Design review of the part built by this model. Coordinates are the model's own, in mm. Face numbers are marked on the shaded views. A direction names the side the tool comes from. Round coordinates to 2 decimals unless told otherwise and drop trailing zeros. Write each loop counter-clockwise with the first axis right and the second up, starting at its lowest first coordinate (ties: lowest second). Pieces come first, ordered by that corner, then holes. Notation, with made-up numbers: M 61,8.5 L 71,8.5 A23 cw 71,32.5 Z; hole C 83,-37 d3. An arc over 180 degrees is marked long. Use CSV: the item, a comma, the result in double quotes.
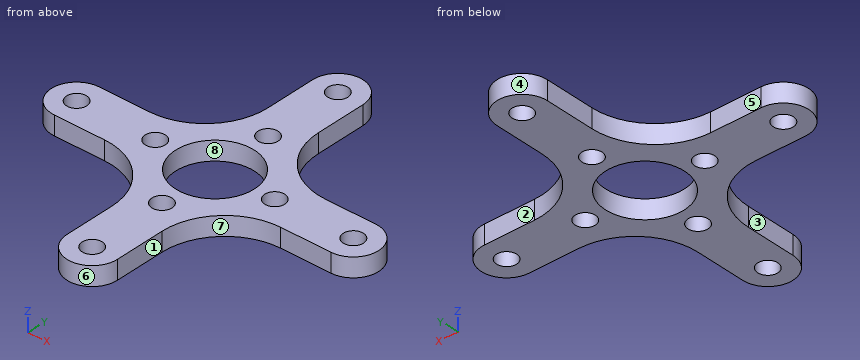
from build123d import *

# Parameters (mm, degrees)
SKETCH_1_R      = 6.25
SKETCH_1_R_2    = 1.6
EXTRUDE_1_DEPTH = 1.5


with BuildPart() as part:
    # Эскиз1 → Бобышка-Вытянуть1 (new body, symmetric)
    with BuildSketch(Plane.XY):
        with BuildLine():
            Line((-22, 4), (-14, 4))
            ThreePointArc((-14, 4), (-6.928932188, 6.928932188), (-4, 14))
            Line((-4, 14), (-4, 22))
            ThreePointArc((-4, 22), (0, 26), (4, 22))
            Line((4, 22), (4, 14))
            ThreePointArc((4, 14), (6.928932188, 6.928932188), (14, 4))
            Line((14, 4), (22, 4))
            ThreePointArc((22, 4), (26, 0), (22, -4))
            Line((22, -4), (14, -4))
            ThreePointArc((14, -4), (6.928932188, -6.928932188), (4, -14))
            Line((4, -14), (4, -22))
            ThreePointArc((4, -22), (0, -26), (-4, -22))
            Line((-4, -22), (-4, -14))
            ThreePointArc((-4, -14), (-6.928932188, -6.928932188), (-14, -4))
            Line((-14, -4), (-22, -4))
            ThreePointArc((-22, -4), (-26, 0), (-22, 4))
        make_face()
        Circle(SKETCH_1_R, mode=Mode.SUBTRACT)
        with Locations((-9.5, 0)):
            Circle(SKETCH_1_R_2, mode=Mode.SUBTRACT)
        with Locations((-22, 0)):
            Circle(SKETCH_1_R_2, mode=Mode.SUBTRACT)
        with Locations((0, 9.5)):
            Circle(SKETCH_1_R_2, mode=Mode.SUBTRACT)
        with Locations((0, 22)):
            Circle(SKETCH_1_R_2, mode=Mode.SUBTRACT)
        with Locations((9.5, 0)):
            Circle(SKETCH_1_R_2, mode=Mode.SUBTRACT)
        with Locations((22, 0)):
            Circle(SKETCH_1_R_2, mode=Mode.SUBTRACT)
        with Locations((0, -22)):
            Circle(SKETCH_1_R_2, mode=Mode.SUBTRACT)
        with Locations((0, -9.5)):
            Circle(SKETCH_1_R_2, mode=Mode.SUBTRACT)
    extrude(amount=EXTRUDE_1_DEPTH, both=True)


solid = part.part
1) Add section C-C on y = 9.5. Write out the cut boundary in (x, z), then the cut area to 3 significant figures.
Answers:
outline,"M -5.07,-1.5 L -1.6,-1.5 L -1.6,1.5 L -5.07,1.5 Z; M 1.6,-1.5 L 5.07,-1.5 L 5.07,1.5 L 1.6,1.5 Z"
area,"20.8 mm²"
2) Wall thickness on line 1 along Y through (x, z) = (0, -0.6); line 2 along Y through (x, z) = (-22, 1.4); line 3 along X through (y, z) = (-1, -0.8): over which ranges is each line inside the solid? List them lowest first. Write a range as [from, to].
Answers:
line 1,"[-26, -23.6], [-20.4, -11.1], [-7.9, -6.25], [6.25, 7.9], [11.1, 20.4], [23.6, 26]"
line 2,"[-4, -1.6], [1.6, 4]"
line 3,"[-25.87, -23.25], [-20.75, -10.75], [-8.25, -6.17], [6.17, 8.25], [10.75, 20.75], [23.25, 25.87]"
3) Add section D-D on x = -9. Write out the cut boundary in (y, z), then the cut area to 3 significant figures.
Answers:
outline,"M -5.34,-1.5 L -1.52,-1.5 L -1.52,1.5 L -5.34,1.5 Z; M 1.52,-1.5 L 5.34,-1.5 L 5.34,1.5 L 1.52,1.5 Z"
area,"22.9 mm²"
4) Machinability: for the marked faces 1, 2, 3, 4 and 5, which of the approach directions +Z, -Z, +X, -X, +Y, -Y give a long, thin tool a straight path to every point of the face, cutting with its end or side? Answer none if there is none.
Answers:
face 1,"+Z, -Z, +X, -Y"
face 2,"+Z, -Z, +X, +Y"
face 3,"+Z, -Z, -X, -Y"
face 4,"+Z, -Z, +Y"
face 5,"+Z, -Z, -X, +Y"
5) Add section B-B on z = -0.7. Give the number of separate pieces and of enclosed holes in the cut face, then the cut area to 3 significant figures.
Answers:
separate pieces,"1"
enclosed holes,"9"
area,"639 mm²"
6) For pin 1 Ø1.5 at (y, z) = (-17, 0) entering from +X; pin 2 Ø0.9 at (y, z) = (16, 0) entering from -X; pin 3 Ø1.5 at (x, z) = (16.5, 0) entering from +Y; pin 4 Ø3 at (x, y) = (9.5, 0) entering from +Z (3 decimals), all flat-tipped, find the tip position at first contact; note any pin that passes through.
Answers:
pin 1,"x = 4"
pin 2,"x = -4"
pin 3,"y = 4"
pin 4,"through"
7) The part is to be moulded in two halves that separate along X. For the marked faces 6, 7 and 8, say which applies: released by +X, released by -X, zero draft, split by the parting line, or undercut.
Answers:
face 6,"split by the parting line"
face 7,"released by +X"
face 8,"undercut"
8) Add section A-A on x = 0. Write out the cut boundary in (y, z), then the cut area to 3 significant figures.
Answers:
outline,"M -26,-1.5 L -23.6,-1.5 L -23.6,1.5 L -26,1.5 Z; M -20.4,-1.5 L -11.1,-1.5 L -11.1,1.5 L -20.4,1.5 Z; M -7.9,-1.5 L -6.25,-1.5 L -6.25,1.5 L -7.9,1.5 Z; M 6.25,-1.5 L 7.9,-1.5 L 7.9,1.5 L 6.25,1.5 Z; M 11.1,-1.5 L 20.4,-1.5 L 20.4,1.5 L 11.1,1.5 Z; M 23.6,-1.5 L 26,-1.5 L 26,1.5 L 23.6,1.5 Z"
area,"80.1 mm²"
